Input: dimensioned drawing with shaded views. Units: mm. Origin: part minimum x, y, z. Round coordinates to 2 decimals unless told otherwise and drop trailing zeros. Write each loop counter-clockwise with the first axis right and the second up, starting at its lowest first coordinate (ties: lowest second). Pieces come first, ordered by that corner, then holes. Notation, with made-up numbers: (-8.75, -9) - (16.25, -9) arc R13 cw to (16.25, 5) - close; hole circle Ø7 at (51.25, 24.25). An arc over 180 degrees is marked (long way). Use one line per item in the form item = value.
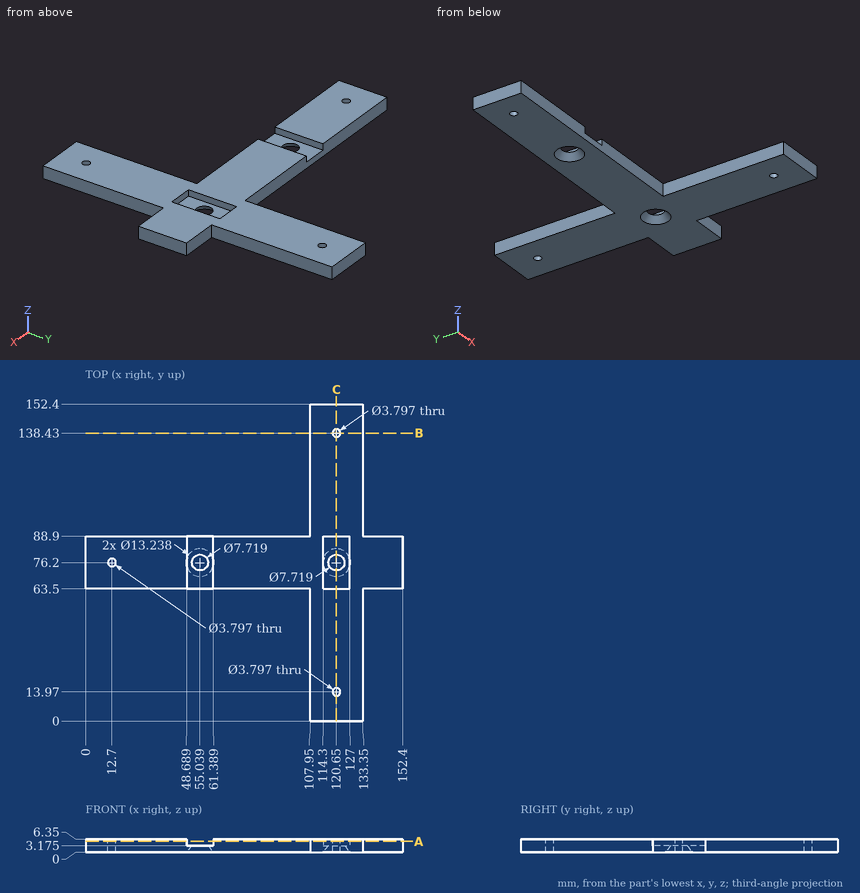
(1) Cut plane C-C on x = 120.65. Count the separate pieces of the cut face and the enclosed holes in it.
Derived:
separate_pieces = 4
enclosed_holes = 0
(2) Cut plane B-B on y = 138.43. Output: boundary loops of the cut face in (x, z), then the cut area to 3 significant figures.
Derived:
outline = (107.95, 0) - (118.75, 0) - (118.75, 6.35) - (107.95, 6.35) - close; (122.55, 0) - (133.35, 0) - (133.35, 6.35) - (122.55, 6.35) - close
area = 137 mm^2
(3) First-contact query: pin 1 Ø1.5 at (y, z) = (39, 3) entering from -X; pin 2 Ø3 at (y, z) = (109, 2.5) entering from +X; pin 3 Ø3 at (x, z) = (141, 2.5) entering from -Y; pin 4 Ø3 at (x, y) = (120.65, 13.97) entering from -Z. Flat tips, straight axial feed; report the tip coordinate or a pass-through.
Derived:
pin_1 = 107.95
pin_2 = 133.35
pin_3 = 63.5
pin_4 = through
(4) Cut plane A-A on z = 5.25. Output: boundary loops of the cut face in (x, y), then the cut area to 3 significant figures.
Derived:
outline = (0, 63.5) - (48.69, 63.5) - (48.69, 88.9) - (0, 88.9) - close; (61.39, 63.5) - (107.95, 63.5) - (107.95, 0) - (133.35, 0) - (133.35, 63.5) - (152.4, 63.5) - (152.4, 88.9) - (133.35, 88.9) - (133.35, 152.4) - (107.95, 152.4) - (107.95, 88.9) - (61.39, 88.9) - close; hole circle Ø3.8 at (12.7, 76.2); hole (114.3, 63.5) - (127, 63.5) - (127, 88.9) - (114.3, 88.9) - close; hole circle Ø3.8 at (120.65, 13.97); hole circle Ø3.8 at (120.65, 138.43)
area = 6,420 mm^2
(5) Material intervals for L1, parallel to X at y = 76.2, z = 5; L2, parallel to Y at x = 120.65, z = 3.25; L3, parallel to X at y = 138.43, z = 3, sorted ascending.
Derived:
L1 = 0 to 10.8, 14.6 to 48.69, 61.39 to 114.3, 127 to 152.4
L2 = 0 to 12.07, 15.87 to 63.5, 88.9 to 136.53, 140.33 to 152.4
L3 = 107.95 to 118.75, 122.55 to 133.35
